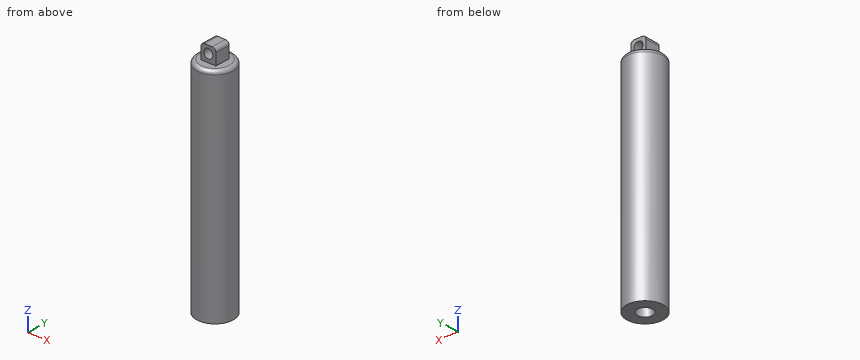
from build123d import *

# Parameters (mm, degrees)
F0_R     = 38.1
F1_DEPTH = 457.2
F2_W     = 31.75
F2_H     = 63.5
F2_R     = 9.525
F3_DEPTH = 15.875
F4_R     = 7.62
F5_R     = 15.875
F6_DEPTH = 450.85


with BuildPart() as f1:
    # F0 (on Top) → F1 (new body)
    with BuildSketch(Plane.XY):
        Circle(F0_R)
    extrude(amount=-F1_DEPTH)

    # F2 (on Front) → F3 (join, symmetric)
    with BuildSketch(Plane.XZ):
        Rectangle(F2_W, F2_H)
        with Locations((0, 16.3000393659)):
            Circle(F2_R, mode=Mode.SUBTRACT)
    extrude(amount=F3_DEPTH, both=True)

    # F4
    f4_edges = [f1.edges().sort_by_distance(p)[0] for p in [
        (15.875, 0, 31.75),
        (-15.875, 0, 31.75),
        (-38.1, 0, 0),
    ]]
    fillet(f4_edges, radius=F4_R)

    # F5 (on face) → F6 (cut)
    with BuildSketch(Plane(origin=(0, 0, -457.2), x_dir=(1, 0, 0), z_dir=(0, 0, -1))):
        Circle(F5_R)
    extrude(amount=-F6_DEPTH, mode=Mode.SUBTRACT)


solid = f1.part
Geometry: final body of the model. Coordinates: model frame, mm. Round coordinates to 2 decimals unless told otherwise and drop trailing zeros. Loops run counter-clockwise (first coordinate to the right, second up) from the corner with the lowest first, then second, coordinate; pieces in that order, holes last. Notation, with made-up numbers: M 8,41 L 45,41 A29 ccw 45,74 Z; hole C 5.5,5.25 d1. An arc over 180 degrees is marked long. Put each result on its own line as item: value. Start each with the question number.
(1) Material intervals for line 1 along X through (y, z) = (-1, -72); line 2 along X through (y, z) = (0.5, -173); line 3 along Y through (x, z) = (0, -208) (3 decimals), sorted ascending. Write a range as [from, to].
(2) Section query B-B (y = 0). Return loops of the section in (x, z) (3 decimals).
(3) Section query A-A (x = 0). Return loops of the section in (y, z) (3 decimals).
(4) Contact query for flat-ended pins moving along their axis: pin 1 Ø12 at (y, z) = (4, 12) entering from +X (3 decimals); pin 2 Ø12 at (x, z) = (-22.5, -39.5) entering from +Y; pin 3 Ø2 at (x, y) = (10, 1.5) entering from +Z. Output: stop coordinate, or through.
(5) Section query C-C (z = -129.5). Return loops of the section in (x, y) (3 decimals).
Findings below:
1. line 1: x = [-38.09, -15.84], [15.84, 38.09]
1. line 2: x = [-38.1, -15.87], [15.87, 38.1]
1. line 3: y = [-38.1, -15.875], [15.875, 38.1]
2. outline: M -38.1,-457.2 L -15.875,-457.2 L -15.875,-6.35 L 15.875,-6.35 L 15.875,-457.2 L 38.1,-457.2 L 38.1,-7.62 A7.62 ccw 30.48,0 L 15.875,0 L 15.875,24.13 A7.62 ccw 8.255,31.75 L -8.255,31.75 A7.62 ccw -15.875,24.13 L -15.875,0 L -30.48,0 A7.62 ccw -38.1,-7.62 Z; hole C 0,16.3 d19.05
3. outline: M -38.1,-457.2 L -15.875,-457.2 L -15.875,-6.35 L 15.875,-6.35 L 15.875,-457.2 L 38.1,-457.2 L 38.1,-7.62 A7.62 ccw 30.48,0 L 15.875,0 L 15.875,6.775 L -15.875,6.775 L -15.875,0 L -30.48,0 A7.62 ccw -38.1,-7.62 Z; M -15.875,25.825 L 15.875,25.825 L 15.875,31.75 L -15.875,31.75 Z
4. pin 1: stops at x = 15.875
4. pin 2: stops at y = 34.34
4. pin 3: stops at z = 31.71
5. outline: C 0,0 d76.2; hole C 0,0 d31.75
